```python
from build123d import *
from build123d.topology import SkipClean

# Parameters (mm, degrees)
REVOLVE_2_ANGLE           = 90
REVOLVE_2_OTHER_WAY_ANGLE = 90
SKETCH_2_R                = 10
CUT_EXTRUDE_1_DEPTH       = 31


with BuildPart() as part:
    # Sketch 1 → Revolve 1 (revolve)
    with BuildSketch(Plane.XY, mode=Mode.PRIVATE) as revolve_1_sk:
        Polygon((15, 30), (15, 0), (20, 0), (20, 50), (15, 50), align=None)
    revolve(revolve_1_sk.sketch.rotate(Axis((0, 50, 0), (0, -1, 0)), 90), axis=Axis((0, 50, 0), (0, -1, 0)))

    # Sketch 1_3 → Revolve 2 (revolve)
    with BuildSketch(Plane.XY):
        with BuildLine():
            Line((0, 30), (0, 50))
            Line((0, 50), (-480, 50))
            ThreePointArc((-480, 50), (-485.857864376, 35.857864376), (-500, 30))
            Line((-500, 30), (0, 30))
        make_face()
    revolve(axis=Axis((0, 50, 0), (-1, 0, 0)), revolution_arc=REVOLVE_2_ANGLE)

    # Sketch 1_3 → Revolve 2 other way (revolve)
    with SkipClean():  # the faces are left unmerged after this step: merging them gives an invalid solid
        with BuildSketch(Plane.XY):
            with BuildLine():
                Line((0, 30), (0, 50))
                Line((0, 50), (-480, 50))
                ThreePointArc((-480, 50), (-485.857864376, 35.857864376), (-500, 30))
                Line((-500, 30), (0, 30))
            make_face()
        revolve(axis=Axis((0, 50, 0), (1, 0, 0)), revolution_arc=REVOLVE_2_OTHER_WAY_ANGLE)

    # Sketch 1_5 → Revolve 4 (revolve)
    with BuildSketch(Plane.XY):
        with BuildLine():
            Line((-500, 50), (-500, 30))
            ThreePointArc((-500, 30), (-485.857864376, 35.857864376), (-480, 50))
            Line((-480, 50), (-500, 50))
        make_face()
    revolve(axis=Axis((-500, 50, 0), (0, -1, 0)))

    # Sketch 2 → Cut-Extrude 1 (cut)
    with BuildSketch(Plane(origin=(0, 50, 0), x_dir=(1, 0, 0), z_dir=(0, 1, 0))):
        with Locations(Location((-500, 0, 0), (0, 0, 270))):
            Circle(SKETCH_2_R)
    extrude(amount=-CUT_EXTRUDE_1_DEPTH, mode=Mode.SUBTRACT)


solid = part.part
```
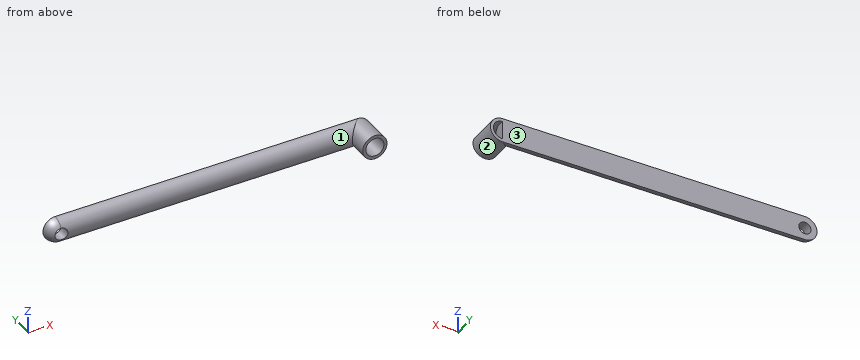
Geometry check sheet. Reference: the model listing, model coordinates, mm. Face numbers are marked on the shaded views. A direction names the side the tool comes from. Coordinates: 2 decimals unless noted, no trailing zeros. Write each loop counter-clockwise with the first axis right and the second up, starting at its lowest first coordinate (ties: lowest second). Pieces come first, ordered by that corner, then holes. Notation, with made-up numbers: (58.25, -20) -> (108.25, -20) arc R28 ccw to (108.25, 4) -> close; hole circle Ø1 at (39, -29). An arc over 180 degrees is marked (long way). Use CSV: the item, a comma, the result in double quotes. Start each with the question number.
Item 1: Cross-section at B-B, the plane y = 14. Record the cut outline in (x, z).
Item 2: Depth check by flat-ended pin: pin 1 Ø8 at (x, y) = (-399, 31.5) entering from -Z (3 decimals); pin 2 Ø10 at (y, z) = (32.5, -2.5) entering from -X; pin 3 Ø22 at (y, z) = (37, -7) entering from +X. Enter the tip coordinate at first touch or a pass-through.
Item 3: Set-up check for the marked faces 1, 2 and 3: record each of +Z, -Z, +X, -X, +Y, -Y from which the full face is reachable in a straight line by a thin tool's end or side.
Item 4: Thickness scan on line 1 (X direction, y = 39, z = 0); line 2 (X direction, y = 36.5, z = 0); line 3 (Y direction, x = -225, z = -1). Record the ranges inside material, lowest first.
Item 5: Cross-section at A-A, the plane z = 0. Record the cut outline in (x, y), plus the area to 3 significant figures.
Item 6: Cross-section at C-C, the plane x = -356.5. Record the cut outline in (y, z), plus the area to 3 significant figures.
Answers:
1,outline,"circle Ø40 at (0, 0); hole circle Ø30 at (0, 0)"
2,pin 1,"z = -13.775"
2,pin 2,"x = -515.47"
2,pin 3,"x = 20"
3,face 1,"-X, -Y"
3,face 2,"-Y"
3,face 3,"+Z, -Z, +X, -X, +Y"
4,line 1,"-516.7 to -510, -490 to 0, 15 to 20"
4,line 2,"-514.76 to -510, -490 to 0, 15 to 20"
4,line 3,"30.03 to 50"
5,outline,"(-520, 50) arc R20 ccw to (-510, 32.68) -> (-510, 50) -> close; (-490, 30) -> (-20, 30) -> (-20, 0) -> (-15, 0) -> (-15, 30) -> (0, 30) -> (0, 50) -> (-490, 50) -> close; (15, 0) -> (20, 0) -> (20, 50) -> (15, 50) -> close"
5,area,"10,300 mm^2"
6,outline,"(50, -20) -> (50, 20) arc R20 ccw to start"
6,area,"628 mm^2"
